Part model, mm, in its own coordinate system. Face numbers are marked on the shaded views. A direction names the side the tool comes from. Coordinates: 2 decimals unless noted, no trailing zeros. Order: outer loops, then holes, each group sorted by start corner. A loop starts at its lowest first (then second) coordinate and runs counter-clockwise, first axis right, second up.
1) Cut at A-A (x = 88.9). List the corners of the cut face in (y, z).
2) Cut at B-B (y = 38.1). List the corners of the cut face in (x, z), and give its area (3 significant figures).
3) Cut at C-C (x = 51.5). List the corners of the cut face in (y, z).
4) Tool access for the marked faces 1 and 2: list every direction of +Z, -Z, +X, -X, +Y, -Y with a clear straight run to the whole face (end or side of a thin tool).
5) Cut at D-D (z = 14). List the corners of the cut face in (x, y).
6) Wall check: L1, parallel to Z at x = 44, y = 45; L2, parallel to Y at x = 43.5, z = 17; L3, parallel to Y at x = 50.8, z = -1.8. Give the ranges that are in metal, low to high.
7) Pin check, flat tips, straight feed: pin 1 Ø10 at (x, z) = (62, 14) entering from +Y; pin 2 Ø6 at (x, y) = (58, 26.5) entering from +Z. Stop position of each tip, or through.
```python
from build123d import *

# Parameters (mm, degrees)
BASE_FLANGE1_DEPTH           = 2.65684
EDGE_FLANGE1_STRIP_W         = 15.94104
EDGE_FLANGE1_STRIP_H         = 2.65684
EDGE_FLANGE1_STRIP_CUT_DEPTH = 101.6
EDGE_FLANGE1_DEPTH           = 101.6
FILLET1_R                    = 6.35
F_10_0_1935_DIAMETER_HOLE1_D = 4.9149
F_1_4_CLEARANCE_HOLE1_D      = 6.7564


# Sheet-metal steps are written as plain solids
with BuildPart() as part:
    # Sketch1 → Base-Flange1 (new body)
    with BuildSketch(Plane.XY):
        Polygon((0, 0), (0, 12.7), (31.75, 50.8), (69.85, 50.8), (101.6, 12.7), (101.6, 0), align=None)
    extrude(amount=-BASE_FLANGE1_DEPTH)

    # Edge-Flange1 strip (across the edge) → Edge-Flange1 strip cut (cut)
    with BuildSketch(Plane.YZ):
        with Locations((-2.65684, -1.32842)):
            Rectangle(EDGE_FLANGE1_STRIP_W, EDGE_FLANGE1_STRIP_H)
    extrude(amount=EDGE_FLANGE1_STRIP_CUT_DEPTH, mode=Mode.SUBTRACT)

    # Edge-Flange1 section (across the edge) → Edge-Flange1 (add)
    with BuildSketch(Plane.YZ):
        with BuildLine():
            Line((0, 2.65684), (0, 22.74316))
            Line((0, 22.74316), (2.65684, 22.74316))
            Line((2.65684, 22.74316), (2.65684, 2.65684))
            ThreePointArc((2.65684, 2.65684), (3.435010419, 0.778170419), (5.31368, 0))
            Line((5.31368, 0), (5.31368, -2.65684))
            ThreePointArc((5.31368, -2.65684), (1.556340839, -1.100499161), (0, 2.65684))
        make_face()
    extrude(amount=EDGE_FLANGE1_DEPTH)

    # Fillet1
    fillet1_edges = [part.edges().sort_by_distance(p)[0] for p in [
        (0, 12.7, -1.32842),
        (31.75, 50.8, -1.32842),
        (69.85, 50.8, -1.32842),
        (101.6, 12.7, -1.32842),
        (0, 1.32842, 22.74316),
        (101.6, 1.32842, 22.74316),
    ]]
    fillet(fillet1_edges, radius=FILLET1_R)

    # #10 (0.1935) Diameter Hole1 (through all)
    with Locations(Plane(origin=(0, 0, 0), x_dir=(-1, 0, 0), z_dir=(0, -1, 0))):
        with Locations((-88.9, -10.04316), (-50.8, -10.04316), (-12.7, -10.04316)):
            Hole(F_10_0_1935_DIAMETER_HOLE1_D / 2)

    # 1/4 Clearance Hole1 (through all)
    with Locations(Plane.XY):
        with Locations((50.8, 38.1)):
            Hole(F_1_4_CLEARANCE_HOLE1_D / 2)


solid = part.part
```
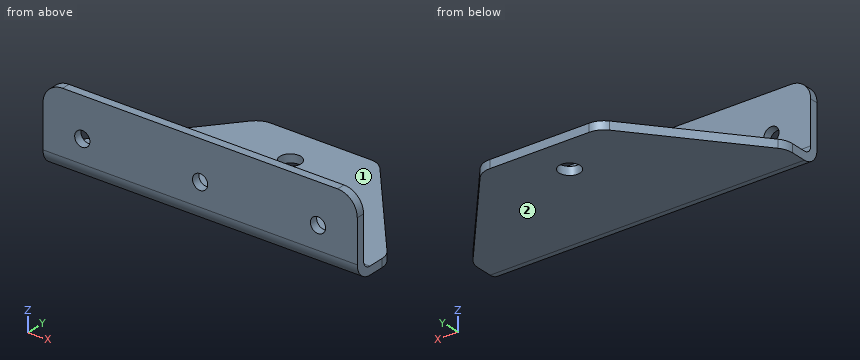
Geometry check:
1. outline: (0, 2.66) arc R5.31 ccw to (5.31, -2.66) - (27.94, -2.66) - (27.94, 0) - (5.31, 0) arc R2.66 cw to (2.66, 2.66) - (2.66, 7.59) - (0, 7.59) - close; (0, 12.5) - (2.66, 12.5) - (2.66, 22.74) - (0, 22.74) - close
2. outline: (21.17, -2.66) - (47.42, -2.66) - (47.42, 0) - (21.17, 0) - close; (54.18, -2.66) - (80.43, -2.66) - (80.43, 0) - (54.18, 0) - close
2. area: 140 mm2
3. outline: (0, 2.66) arc R5.31 ccw to (5.31, -2.66) - (34.8, -2.66) - (34.8, 0) - (5.31, 0) arc R2.66 cw to (2.66, 2.66) - (2.66, 7.69) - (0, 7.69) - close; (0, 12.4) - (2.66, 12.4) - (2.66, 22.74) - (0, 22.74) - close; (41.4, -2.66) - (50.8, -2.66) - (50.8, 0) - (41.4, 0) - close
4. face 1: +Z, +X, -X, +Y
4. face 2: -Z, +X, -X, +Y, -Y
5. outline: (0, 0) - (101.6, 0) - (101.6, 2.66) - (0, 2.66) - close
6. L1: z = -2.66 to 0
6. L2: y = 0 to 2.66
6. L3: y = 2.42 to 34.72, 41.48 to 50.8
7. pin 1: stops at y = 2.66
7. pin 2: stops at z = 0
